For this review, take the finished solid that the model builds, in its own axes (mm). A direction names the side the tool comes from. Coordinates: 2 decimals unless noted, no trailing zeros. Loops run counter-clockwise (first coordinate to the right, second up) from the corner with the lowest first, then second, coordinate; pieces in that order, holes last. Notation, with made-up numbers: (-6.5, 29.5) -> (38.5, 29.5) arc R28 ccw to (38.5, 49.5) -> close; hole circle Ø1 at (0.25, 64.25). An arc over 180 degrees is marked (long way). Answer in a Markdown table with one row per item.
from build123d import *

# Parameters (mm, degrees)
F0_W     = 57.912
F0_H     = 74.5998
F1_DEPTH = 7.493
F2_R     = 7.366
F3_R     = 1.27
F4_R     = 2.54


with BuildPart() as f1:
    # F0 (on Top) → F1 (new body)
    with BuildSketch(Plane.XY):
        with Locations((20.296287, 12.616272)):
            Rectangle(F0_W, F0_H)
        with BuildLine():
            ThreePointArc((17.756287, 3.632269), (8.054824, 8.929138), (3.925598, 19.182172))
            Line((3.925598, 19.182172), (2.655598, 19.182172))
            Line((2.655598, 19.182172), (2.655598, 20.452172))
            Line((2.655598, 20.452172), (3.925598, 20.452172))
            ThreePointArc((3.925598, 20.452172), (8.054824, 30.705205), (17.756287, 36.002075))
            Line((17.756287, 36.002075), (17.756287, 38.034075))
            Line((17.756287, 38.034075), (22.836287, 38.034075))
            Line((22.836287, 38.034075), (22.836287, 36.002075))
            ThreePointArc((22.836287, 36.002075), (36.679287, 19.817172), (22.836287, 3.632269))
            Line((22.836287, 3.632269), (22.836287, 0.153448))
            Line((22.836287, 0.153448), (17.756287, 0.153448))
            Line((17.756287, 0.153448), (17.756287, 3.632269))
        make_face(mode=Mode.SUBTRACT)
    extrude(amount=F1_DEPTH)

    # F2
    f2_edges = [f1.edges().sort_by_distance(p)[0] for p in [
        (-8.659713, -24.683628, 3.7465),
        (49.252287, -24.683628, 3.7465),
        (49.252287, 49.916172, 3.7465),
        (-8.659713, 49.916172, 3.7465),
    ]]
    fillet(f2_edges, radius=F2_R)

    # F3
    f3_edges = [f1.edges().sort_by_distance(p)[0] for p in [
        (-8.659713, 12.616272, 7.493),
    ]]
    fillet(f3_edges, radius=F3_R)

    # F4
    f4_edges = [f1.edges().sort_by_distance(p)[0] for p in [
        (-8.659713, 12.616272, 0),
    ]]
    fillet(f4_edges, radius=F4_R)


solid = f1.part
Item 1: Take a section at C-C, the plane y = 33. State the section outline as (x, z) points.
Worked answers:
| item | result |
|---|---|
| outline | (-8.66, 2.54) arc R2.54 ccw to (-6.12, 0) -> (10.57, 0) -> (10.57, 7.49) -> (-7.39, 7.49) arc R1.27 ccw to (-8.66, 6.22) -> close; (30.02, 0) -> (46.71, 0) arc R2.54 ccw to (49.25, 2.54) -> (49.25, 6.22) arc R1.27 ccw to (47.98, 7.49) -> (30.02, 7.49) -> close |
Item 2: The part is to be moulded in two halves that separate along X. For faces 1 (the flat face through (17.756, 2, 4)), 2 (the cylindrical face through (48.528, 12.197, 0.764)), 3 (the flat face through (32, 5, 0)), say which applies: +X half, -X half, draft (parallel to the pull), parting line (faces both ways), or undercut.
Worked answers:
| item | result |
|---|---|
| face 1 | undercut |
| face 2 | +X half |
| face 3 | draft |
Item 3: For L1, parallel to Y at x = 19.5, z = 5.5; L2, parallel to X at y = 17, z = 6; L3, parallel to Y at x = 9.5, z = 2.5, list the stretches that pass through material, from the lowest coordinate up.
Worked answers:
| item | result |
|---|---|
| L1 | -24.68 to 0.15, 38.03 to 49.92 |
| L2 | -8.66 to 4.16, 36.44 to 49.25 |
| L3 | -24.68 to 7.49, 32.14 to 49.92 |
Item 4: Take a section at A-A, the plane x = 20. State the section outline as (y, z) points.
Worked answers:
| item | result |
|---|---|
| outline | (-24.68, 2.54) arc R2.54 ccw to (-22.14, 0) -> (0.15, 0) -> (0.15, 7.49) -> (-23.41, 7.49) arc R1.27 ccw to (-24.68, 6.22) -> close; (38.03, 0) -> (47.38, 0) arc R2.54 ccw to (49.92, 2.54) -> (49.92, 6.22) arc R1.27 ccw to (48.65, 7.49) -> (38.03, 7.49) -> close |
Item 5: For faces 4 (the cylindrical face through (8.16, 8.81, 3.69)), 5 (the flat face through (20, -24.684, 4)), list the 3-axis set-ups (+Z, -Z, +X, -X, +Y, -Y) from which the entire face can be reached by the end or side of a thin tool; tool diameter is ignored.
Worked answers:
| item | result |
|---|---|
| face 4 | +Z, -Z |
| face 5 | +Z, -Z, +X, -X, -Y |
Item 6: Take a section at B-B, the plane z = 3.75. State the section outline as (x, y) points, and give its area (3 significant figures).
Worked answers:
| item | result |
|---|---|
| outline | (-8.66, -17.32) arc R7.37 ccw to (-1.29, -24.68) -> (41.89, -24.68) arc R7.37 ccw to (49.25, -17.32) -> (49.25, 42.55) arc R7.37 ccw to (41.89, 49.92) -> (-1.29, 49.92) arc R7.37 ccw to (-8.66, 42.55) -> close; hole (2.66, 19.18) -> (3.93, 19.18) arc R16.38 ccw to (17.76, 3.63) -> (17.76, 0.15) -> (22.84, 0.15) -> (22.84, 3.63) arc R16.38 ccw to (22.84, 36) -> (22.84, 38.03) -> (17.76, 38.03) -> (17.76, 36) arc R16.38 ccw to (3.93, 20.45) -> (2.66, 20.45) -> close |
| area | 3,400 mm² |
Item 7: Insertion check: pin 1 (0.6 mm diameter, centred on y = 20, z = 2, fed in from +X). The pin has a flat end and moves straight along its axis. Give the tip position at first contact, or say it passes through.
Worked answers:
| item | result |
|---|---|
| pin 1 | x = 49.24 |
